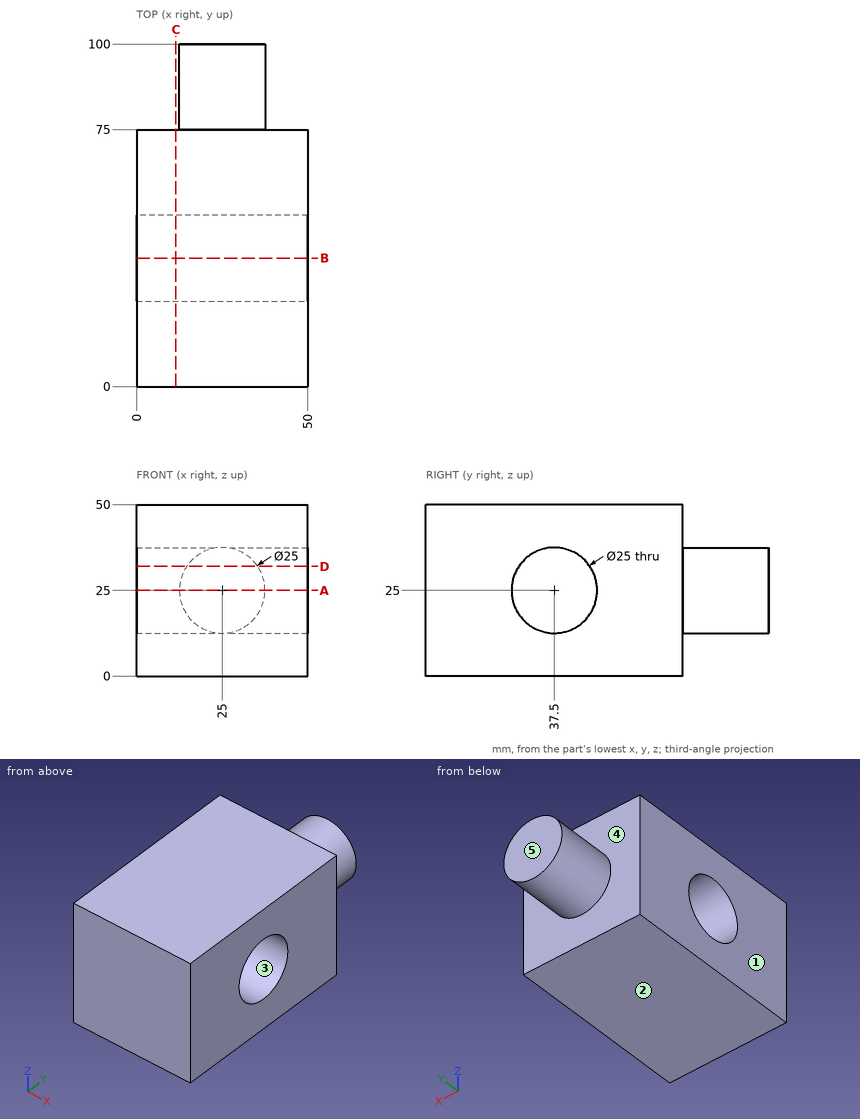
Geometry: see drawing. Coordinates: mm, zero at the bounding-box minimum. A direction names the side the tool comes from. Give positions to 0.01 mm unless a question says otherwise; leave off trailing zeros. Loops run counter-clockwise (first coordinate to the right, second up) from the corner with the lowest first, then second, coordinate; pieces in that order, holes last. Notation, with made-up numbers: (76.25, -15) - (85.25, -15) arc R36 cw to (85.25, 21) - close; hole circle Ø2 at (44, 12.25). An arc over 180 degrees is marked (long way). Use CSV: the item, a comma, the result in double quotes. Start each with the question number.
Item 1: Contact query for a flat-ended pin moving along its axis: P1, Ø6, axis at x = 27, z = 9, coming from the +Y side. Output: stop coordinate, or through.
Item 2: Line query: line 1 (Z direction, x = 13, y = 37.5); line 2 (Y direction, x = 23, z = 28.5); line 3 (Y direction, x = 4, z = 33.5). Output: solid intervals per line, ascending.
Item 3: Section A-A on z = 25. Return loops of the section in (x, y), then the cut area to 4 significant figures.
Item 4: Section C-C on x = 11.5. Return loops of the section in (y, z).
Item 5: Section B-B on y = 37.5. Return loops of the section in (x, z), then the cut area to 3 significant figures.
Item 6: Section D-D on z = 32. Return loops of the section in (x, y).
Item 7: Reachability of the marked faces 4 and 5 from +Z, -Z, +X, -X, +Y, -Y: full face, straight path, thin tool, end or side. Return the list, or none.
Item 8: Mould query, pull axis Z, two halves, no side actions, for the marked faces 1, 2 and 3. Classes: pulls with the +Z half, pulls with the -Z half, needs draft (parallel to the pull), parting line crosses it, or undercut.
Ans:
1,P1,"stops at y = 75"
2,line 1,"z = 0 to 12.5, 37.5 to 50"
2,line 2,"y = 0 to 25.5, 49.5 to 100"
2,line 3,"y = 0 to 28.33, 46.67 to 75"
3,outline,"(0, 0) - (50, 0) - (50, 25) - (0, 25) - close; (0, 50) - (50, 50) - (50, 75) - (37.5, 75) - (37.5, 100) - (12.5, 100) - (12.5, 75) - (0, 75) - close"
3,area,"3,125 mm2"
4,outline,"(0, 0) - (75, 0) - (75, 50) - (0, 50) - close; hole circle Ø25 at (37.5, 25)"
5,outline,"(0, 0) - (50, 0) - (50, 12.5) - (0, 12.5) - close; (0, 37.5) - (50, 37.5) - (50, 50) - (0, 50) - close"
5,area,"1,250 mm2"
6,outline,"(0, 0) - (50, 0) - (50, 27.14) - (0, 27.14) - close; (0, 47.86) - (50, 47.86) - (50, 75) - (35.36, 75) - (35.36, 100) - (14.64, 100) - (14.64, 75) - (0, 75) - close"
7,face 4,"+Y"
7,face 5,"+Z, -Z, +X, -X, +Y"
8,face 1,"needs draft"
8,face 2,"pulls with the -Z half"
8,face 3,"undercut"
